The figure shows three views and two pictorial views of one solid part (mm, origin at its lowest corner). Answer the questions. A direction names the side the tool comes from. Round coordinates to 2 decimals unless told otherwise and drop trailing zeros. Write each loop counter-clockwise with the first axis right and the second up, starting at its lowest first coordinate (ties: lowest second). Pieces come first, ordered by that corner, then holes. Notation, with made-up numbers: (65.5, 4.5) - (108.5, 4.5) arc R17 ccw to (108.5, 29.5) - close; hole circle Ø8 at (57.5, -5). An arc over 180 degrees is marked (long way). Answer as CSV lines item,"result". Start each with the question number.
Item 1: Straight lines are drawn through the part: line 1 along Y through (x, z) = (11, 3.4) (3 decimals); line 2 along Y through (x, z) = (11.75, 2.75); line 3 along Z through (x, y) = (10.75, 21.25). For each, find the intervals that lie inside material, in ascending order. Write a range as [from, to].
Item 2: A cutting plane is placed at D-D on y = 18.25. Determine the outline of the cut face in (x, z).
Item 3: A cutting plane is placed at C-C on z = 11.25. Determine the outline of the cut face in (x, y), and give its area (3 significant figures).
Item 4: For a pull along X with two mould halves and no side action, classify the marked faces 1, 2 and 3 as pulls with the +X half, pulls with the -X half, needs draft (parallel to the pull), parting line crosses it, or undercut.
Item 5: Which of the six approach directions +Z, -Z, +X, -X, +Y, -Y give full straight-line access (tool end or side, diameter ignored) to the marked faces 4 and 5?
Item 6: A cutting plane is placed at A-A on x = 11. Determine the outline of the cut face in (y, z) (3 decimals).
Item 7: Flat-ended cylindrical pins translate along their axes: pin 1 (13 mm diameter, centred on x = 11, y = 11, fed in from +Z); pin 2 (4 mm diameter, centred on y = 19, z = 2, fed in from -X); pin 3 (5.5 mm diameter, centred on x = 19.035, y = 11, fed in from +Z); pin 4 (4 mm diameter, centred on x = 16, z = 10, fed in from -Y). Find the tip coordinate at first contact, or state that the pin passes through.
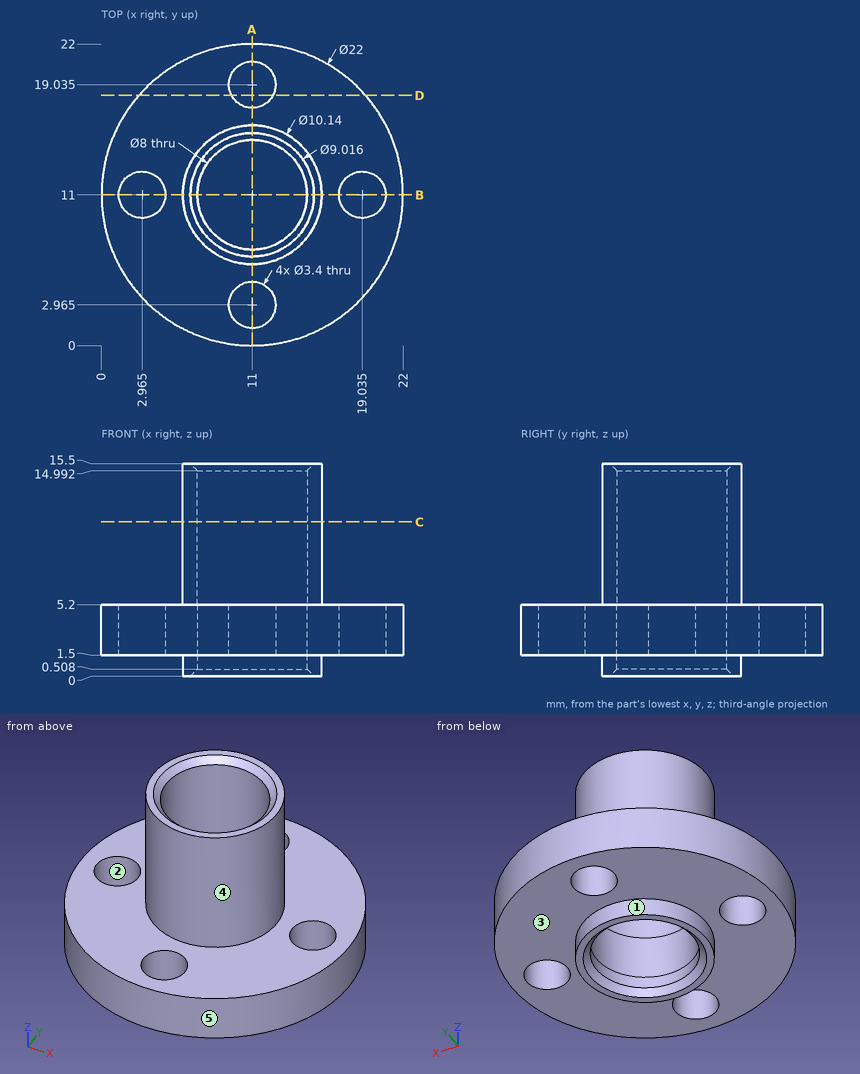
Geometry says:
1,line 1,"y = [0, 1.265], [4.665, 7], [15, 17.335], [20.735, 22]"
1,line 2,"y = [0.03, 1.44], [4.49, 7.07], [14.93, 17.51], [20.56, 21.97]"
1,line 3,"z = [1.5, 5.2]"
2,outline,"(2.73, 1.5) - (9.49, 1.5) - (9.49, 5.2) - (2.73, 5.2) - close; (12.51, 1.5) - (19.27, 1.5) - (19.27, 5.2) - (12.51, 5.2) - close"
3,outline,"circle Ø10.14 at (11, 11); hole circle Ø8 at (11, 11)"
3,area,"30.5 mm^2"
4,face 1,"parting line crosses it"
4,face 2,"undercut"
4,face 3,"needs draft"
5,face 4,"+Z"
5,face 5,"+Z, -Z"
6,outline,"(0, 1.5) - (1.265, 1.5) - (1.265, 5.2) - (0, 5.2) - close; (4.665, 1.5) - (5.93, 1.5) - (5.93, 0) - (6.492, 0) - (7, 0.508) - (7, 14.992) - (6.492, 15.5) - (5.93, 15.5) - (5.93, 5.2) - (4.665, 5.2) - close; (15, 0.508) - (15.508, 0) - (16.07, 0) - (16.07, 1.5) - (17.335, 1.5) - (17.335, 5.2) - (16.07, 5.2) - (16.07, 15.5) - (15.508, 15.5) - (15, 14.992) - close; (20.735, 1.5) - (22, 1.5) - (22, 5.2) - (20.735, 5.2) - close"
7,pin 1,"stops at z = 15.5"
7,pin 2,"stops at x = 1.78"
7,pin 3,"stops at z = 5.2"
7,pin 4,"stops at y = 6.91"
